from build123d import *

# Parameters (mm, degrees)
SKETCH1_R           = 20
BOSS_EXTRUDE1_DEPTH = 1.5
SKETCH2_R           = 15
SKETCH2_R_2         = 13
BOSS_EXTRUDE2_DEPTH = 30
SKETCH3_R           = 10
CUT_EXTRUDE1_DEPTH  = 30


with BuildPart() as part:
    # Sketch1 → Boss-Extrude1 (new body)
    with BuildSketch(Plane.XY):
        Circle(SKETCH1_R)
    extrude(amount=BOSS_EXTRUDE1_DEPTH)

    # Sketch2 → Boss-Extrude2 (add)
    with BuildSketch(Plane.XY.offset(1.5)):
        Circle(SKETCH2_R)
        Circle(SKETCH2_R_2, mode=Mode.SUBTRACT)
    extrude(amount=BOSS_EXTRUDE2_DEPTH)

    # Sketch3 → Cut-Extrude1 (cut)
    with BuildSketch(Plane(origin=(0, 0, 0), x_dir=(-1, 0, 0), z_dir=(0, 0, -1))):
        Circle(SKETCH3_R)
    extrude(amount=-CUT_EXTRUDE1_DEPTH, mode=Mode.SUBTRACT)


solid = part.part
Check sheet for the modelled part. Datum: model origin and axes. Units: mm. A direction names the side the tool comes from. Round coordinates to 2 decimals unless told otherwise and drop trailing zeros. Order: outer loops, then holes, each group sorted by start corner. A loop starts at its lowest first (then second) coordinate and runs counter-clockwise, first axis right, second up.
Q1. Cross-section at A-A, the plane y = 0. Enter the section's corners in (x, z).
Filled sheet:
outline: (-20, 0) - (-10, 0) - (-10, 1.5) - (-13, 1.5) - (-13, 31.5) - (-15, 31.5) - (-15, 1.5) - (-20, 1.5) - close; (10, 0) - (20, 0) - (20, 1.5) - (15, 1.5) - (15, 31.5) - (13, 31.5) - (13, 1.5) - (10, 1.5) - close
Q2. Cross-section at D-D, the plane x = -11. Enter the section's corners in (y, z), plus the area to 3 significant figures.
Filled sheet:
outline: (-16.7, 0) - (16.7, 0) - (16.7, 1.5) - (10.2, 1.5) - (10.2, 31.5) - (6.93, 31.5) - (6.93, 1.5) - (-6.93, 1.5) - (-6.93, 31.5) - (-10.2, 31.5) - (-10.2, 1.5) - (-16.7, 1.5) - close
area: 246 mm2
Q3. Depth check by flat-ended pin: P1, Ø8, axis at x = -4.5, y = -4.5, coming from the +Z side; P2, Ø8, axis at x = -13, z = 24, coming from the -Y side; P3, Ø2, axis at y = 9, z = 4.5, coming from the -X side. Enter the tip coordinate at first touch or a pass-through.
Filled sheet:
P1: stops at z = 1.5
P2: stops at y = -12
P3: stops at x = -12.69
Q4. Set-up check for faces 1 (the face through (2.17, -9.76, 0.74)), 2 (the face through (-14.985, 0.66, 16.29)): record each of +Z, -Z, +X, -X, +Y, -Y from which the full face is reachable in a straight line by a thin tool's end or side.
Filled sheet:
face 1: +Z, -Z
face 2: +Z
Q5. Cross-section at C-C, the plane z = 12.5. Enter the section's corners in (x, y).
Filled sheet:
outline: circle Ø30 at (0, 0); hole circle Ø26 at (0, 0)
Q6. Scan lines: L1, parallel to Y at x = 0, z = 1; L2, parallel to Z at x = 3.5, y = -15; L3, parallel to Y at x = 0, z = 19. Record each from-to range of solid material in increasing order.
Filled sheet:
L1: y = -20 to -10, 10 to 20
L2: z = 0 to 1.5
L3: y = -15 to -13, 13 to 15
Q7. Draft check along Y on faces 3 (the face through (-4.336, -19.524, 0.74)), 4 (the face through (-0.1, 13.4, 31.5)), 5 (the face through (7, -8, 1.5)). Enter one of: pulls with the +Y half, pulls with the -Y half, needs draft (parallel to the pull), parting line crosses it, or undercut.
Filled sheet:
face 3: parting line crosses it
face 4: needs draft
face 5: undercut
